Check sheet for the modelled part. Datum: model origin and axes. Units: mm. A direction names the side the tool comes from. Coordinates: 2 decimals unless noted, no trailing zeros. Use a Markdown table: item, result. Add a question column.
1) Thickness scan on line 1 (Y direction, x = 65.5, z = 6.5); line 2 (X direction, y = 33, z = 2.5) (3 decimals); line 3 (Y direction, x = -7, z = 2.5) (3 decimals). Record the ranges inside material, lowest first.
2) Draft check along X on faces 1 (the flat face through (72.5, -2, 6)), 2 (the flat face through (-47, 2, 0)), 3 (the flat face through (1, 105, 7)). Enter one of: pulls with the +X half, pulls with the -X half, needs draft (parallel to the pull), parting line crosses it, or undercut.
3) Sectioned sample at C-C, the plane z = 7.25. State how many separate pieces and enclosed holes the cut face has, then the cut area to 3 significant figures.
4) Tool access check on faces 4 (the cylindrical face through (43.24, 99.615, 1.732)), 5 (the cylindrical face through (63.42, 51.01, 3.53)), 6 (the cylindrical face through (63.84, 56.52, 7.58)). Record the directions out of +Z, -Z, +X, -X, +Y, -Y that give a thin tool (end or side, any length) a straight path to the whole face; none if there is none.
5) Go/stop test with flat-tipped pins: P1, Ø10, axis at x = 36, y = 122.5, coming from the -Z side; P2, Ø4, axis at x = 37.5, y = -123, coming from the -Z side; P3, Ø1, axis at x = -38, y = 1.5, coming from the +Z side; P4, Ø4.5, axis at x = -37.5, y = -124.5, coming from the -Z side. Record where each tip stops, or that it passes through.
from build123d import *

# Parameters (mm, degrees)
ESBO_O1_W                                           = 145
ESBO_O1_H                                           = 260
RESSALTO_EXTRUS_O1_DEPTH                            = 10
ESBO_O2_W                                           = 145
ESBO_O2_H                                           = 260
CORTE_EXTRUS_O3_DEPTH                               = 2
CORTE_EXTRUS_O4_DEPTH                               = 150.185287478
REBAIXO_PARA_PARAFUSO_COM_CABE_A_PANELA_D           = 4.5
REBAIXO_PARA_PARAFUSO_COM_CABE_A_PANELA_CBORE_D     = 9
REBAIXO_PARA_PARAFUSO_COM_CABE_A_PANELA_CBORE_DEPTH = 3.1
CORTE_EXTRUS_O5_DEPTH                               = 7
ESBO_O4_W                                           = 3.53
ESBO_O4_H                                           = 2.765
ESBO_O13_W                                          = 3.53
ESBO_O13_H                                          = 2.5
FILETE1_R                                           = 20


with BuildPart() as part:
    # Esboço1 → Ressalto-extrusão1 (new body)
    with BuildSketch(Plane.XY):
        Rectangle(ESBO_O1_W, ESBO_O1_H)
    extrude(amount=RESSALTO_EXTRUS_O1_DEPTH)

    # Esboço2 → Corte-extrusão3 (cut)
    with BuildSketch(Plane.XY):
        Rectangle(ESBO_O2_W, ESBO_O2_H)
        with BuildLine():
            Line((-46.5, -110), (46.5, -110))
            ThreePointArc((46.5, -110), (50.742640687, -108.242640687), (52.5, -104))
            Line((52.5, -104), (52.5, 104))
            ThreePointArc((52.5, 104), (50.742640687, 108.242640687), (46.5, 110))
            Line((46.5, 110), (-46.5, 110))
            ThreePointArc((-46.5, 110), (-50.742640687, 108.242640687), (-52.5, 104))
            Line((-52.5, 104), (-52.5, -104))
            ThreePointArc((-52.5, -104), (-50.742640687, -108.242640687), (-46.5, -110))
        make_face(mode=Mode.SUBTRACT)
    extrude(amount=CORTE_EXTRUS_O3_DEPTH, mode=Mode.SUBTRACT)

    # Esboço5 → Corte-extrusão4 (cut, through all)
    with BuildSketch(Plane(origin=(0, 0, 0), x_dir=(-1, 0, 0), z_dir=(0, 0, -1))):
        with BuildLine():
            Line((-34.5, -95), (34.5, -95))
            ThreePointArc((34.5, -95), (36.621320344, -94.121320344), (37.5, -92))
            Line((37.5, -92), (37.5, 92))
            ThreePointArc((37.5, 92), (36.621320344, 94.121320344), (34.5, 95))
            Line((34.5, 95), (-34.5, 95))
            ThreePointArc((-34.5, 95), (-36.621320344, 94.121320344), (-37.5, 92))
            Line((-37.5, 92), (-37.5, -92))
            ThreePointArc((-37.5, -92), (-36.621320344, -94.121320344), (-34.5, -95))
        make_face()
    extrude(amount=-CORTE_EXTRUS_O4_DEPTH, mode=Mode.SUBTRACT)

    # Rebaixo para parafuso com cabeça panela de M41 (through all)
    with Locations(Plane(origin=(0, 0, 2), x_dir=(-1, 0, 0), z_dir=(0, 0, -1))):
        with Locations((-37.5, 123), (37.5, 123), (65.5, 55), (65.5, -55), (37.5, -123), (-37.5, -123), (-65.5, -55), (-65.5, 55)):
            CounterBoreHole(REBAIXO_PARA_PARAFUSO_COM_CABE_A_PANELA_D / 2, REBAIXO_PARA_PARAFUSO_COM_CABE_A_PANELA_CBORE_D / 2, REBAIXO_PARA_PARAFUSO_COM_CABE_A_PANELA_CBORE_DEPTH)

    # Esboço9 → Corte-extrusão5 (cut)
    with BuildSketch(Plane.XY.offset(10)):
        with BuildLine():
            Line((-45, -105), (45, -105))
            ThreePointArc((45, -105), (47.121320344, -104.121320344), (48, -102))
            Line((48, -102), (48, 102))
            ThreePointArc((48, 102), (47.121320344, 104.121320344), (45, 105))
            Line((45, 105), (-45, 105))
            ThreePointArc((-45, 105), (-47.121320344, 104.121320344), (-48, 102))
            Line((-48, 102), (-48, -102))
            ThreePointArc((-48, -102), (-47.121320344, -104.121320344), (-45, -105))
        make_face()
    extrude(amount=-CORTE_EXTRUS_O5_DEPTH, mode=Mode.SUBTRACT)

    # Varredura de corte3: sweep along a path in Esboço14
    with BuildLine(Plane(origin=(0, 0, 2), x_dir=(-1, 0, 0), z_dir=(0, 0, -1))) as varredura_de_corte3_path:
        Line((-47.5, -115), (47.5, -115))
        ThreePointArc((47.5, -115), (54.571067812, -112.071067812), (57.5, -105))
        Line((57.5, -105), (57.5, 105))
        ThreePointArc((57.5, 105), (54.571067812, 112.071067812), (47.5, 115))
        Line((47.5, 115), (-47.5, 115))
        ThreePointArc((-47.5, 115), (-54.571067812, 112.071067812), (-57.5, 105))
        Line((-57.5, 105), (-57.5, -105))
        ThreePointArc((-57.5, -105), (-54.571067812, -112.071067812), (-47.5, -115))
    # Esboço4 → Varredura de corte3 (sweep, cut)
    with BuildSketch(Plane(origin=(0, 0, 0), x_dir=(1, 0, 0), z_dir=(0, 1, 0))):
        with Locations((57.5, -3.3825)):
            Rectangle(ESBO_O4_W, ESBO_O4_H)
    sweep(path=varredura_de_corte3_path.line, mode=Mode.SUBTRACT)

    # Varredura de corte2: sweep along a path in Esboço11
    with BuildLine(Plane.XY.offset(3)) as varredura_de_corte2_path:
        Line((-37.5, -100), (37.5, -100))
        ThreePointArc((37.5, -100), (41.742640687, -98.242640687), (43.5, -94))
        Line((43.5, -94), (43.5, 94))
        ThreePointArc((43.5, 94), (41.742640687, 98.242640687), (37.5, 100))
        Line((37.5, 100), (-37.5, 100))
        ThreePointArc((-37.5, 100), (-41.742640687, 98.242640687), (-43.5, 94))
        Line((-43.5, 94), (-43.5, -94))
        ThreePointArc((-43.5, -94), (-41.742640687, -98.242640687), (-37.5, -100))
    # Esboço13 → Varredura de corte2 (sweep, cut)
    with BuildSketch(Plane(origin=(0, 0, 0), x_dir=(1, 0, 0), z_dir=(0, 1, 0))):
        with Locations((43.765, -1.75)):
            Rectangle(ESBO_O13_W, ESBO_O13_H)
    sweep(path=varredura_de_corte2_path.line, mode=Mode.SUBTRACT)

    # Filete1
    filete1_edges = [part.edges().sort_by_distance(p)[0] for p in [
        (72.5, -130, 6),
        (-72.5, -130, 6),
        (-72.5, 130, 6),
        (72.5, 130, 6),
    ]]
    fillet(filete1_edges, radius=FILETE1_R)


solid = part.part
Solved:
| question | item | result |
|---|---|---|
| 1 | line 1 | y = -125.2 to -57.25, -52.75 to 52.75, 57.25 to 125.2 |
| 1 | line 2 | x = -72.5 to -59.265, -55.735 to -45.53, -42 to -37.5, 37.5 to 42, 45.53 to 55.735, 59.265 to 72.5 |
| 1 | line 3 | y = -130 to -116.765, -113.235 to -102.03, -98.5 to -95, 95 to 98.5, 102.03 to 113.235, 116.765 to 130 |
| 2 | face 1 | pulls with the +X half |
| 2 | face 2 | needs draft |
| 2 | face 3 | undercut |
| 3 | separate pieces | 1 |
| 3 | enclosed holes | 9 |
| 3 | area | 17,100 mm2 |
| 4 | face 4 | +Z |
| 4 | face 5 | -Z |
| 4 | face 6 | +Z, -Z |
| 5 | P1 | stops at z = 2 |
| 5 | P2 | passes through |
| 5 | P3 | stops at z = 3 |
| 5 | P4 | stops at z = 5.1 |
